```python
from build123d import *

# Parameters (mm, degrees)
SKETCH_1_W                = 33
SKETCH_1_H                = 6
EXTRUDE_1_DEPTH           = 30
SKETCH_3_R                = 6
EXTRUDE_2_DEPTH           = 10
SKETCH_4_R                = 3.1
CUT_EXTRUDE_1_DEPTH       = 15
SKETCH_5_R                = 1.75
CUT_EXTRUDE_2_DEPTH       = 48.053161424
EXTRUDE_3_REACH           = 49.381
EXTRUDE_3_END_RADIUS      = 6
SKETCH_10_R               = 1
HOLE_WIZARD_M4_7_D        = 3.3
HOLE_WIZARD_M4_7_DEPTH    = 15
HOLE_WIZARD_M4_7_TIP      = 0.991420021
EXTRUDE_4_REACH           = 49.381
EXTRUDE_4_END_RADIUS      = 6
SKETCH_17_R               = 1.5
HOLE_WIZARD_M4_8_D        = 3.3
HOLE_WIZARD_M4_8_DEPTH    = 13
HOLE_WIZARD_M4_8_TIP      = 0.991420021
HOLE_WIZARD_1_D           = 3.4
HOLE_WIZARD_1_CBORE_D     = 6
HOLE_WIZARD_1_CBORE_DEPTH = 3.4
CUT_EXTRUDE_3_DEPTH       = 46.70557955


with BuildPart() as part:
    # 草图1 → 凸台-拉伸1 (new body)
    with BuildSketch(Plane.XY):
        with Locations((16.5, -3)):
            Rectangle(SKETCH_1_W, SKETCH_1_H)
    extrude(amount=EXTRUDE_1_DEPTH)

    # 草图3 → 凸台-拉伸2 (add)
    with BuildSketch(Plane.XZ.offset(6)):
        with Locations(Location((10.6, 15, 0), (0, 0, 90))):
            Circle(SKETCH_3_R)
    extrude(amount=EXTRUDE_2_DEPTH)

    # 草图4 → 切除-拉伸1 (cut)
    with BuildSketch(Plane.XZ.offset(16)):
        with Locations(Location((10.6, 15, 0), (0, 0, 270))):
            Circle(SKETCH_4_R)
    extrude(amount=-CUT_EXTRUDE_1_DEPTH, mode=Mode.SUBTRACT)

    # 草图5 → 切除-拉伸2 (cut, through all)
    with BuildSketch(Plane.XZ.offset(1)):
        with Locations(Location((10.6, 15, 0), (0, 0, 270))):
            Circle(SKETCH_5_R)
    extrude(amount=-CUT_EXTRUDE_2_DEPTH, mode=Mode.SUBTRACT)

    # 凸台-拉伸3: up to this cylinder (the profile starts outside it)
    extrude_3_end = Plane(origin=(10.6, -11, 15), z_dir=(0, 1, 0)) * Cylinder(EXTRUDE_3_END_RADIUS, 111.762, mode=Mode.PRIVATE)
    # 草图10 → 凸台-拉伸3 (add, up to the surface)
    with BuildSketch(Plane.XY, mode=Mode.PRIVATE) as extrude_3_sk1:
        with Locations(Location((10.6, -11, 0), (0, 0, 180))):
            Circle(SKETCH_10_R)
    extrude_3_tool1 = extrude(extrude_3_sk1.sketch, amount=EXTRUDE_3_REACH, mode=Mode.PRIVATE) - extrude_3_end
    add(extrude_3_tool1.solids().sort_by_distance((10.6, -11, 0))[0])

    # M4 螺纹孔7
    with Locations(Plane(origin=(10.6, -11, 0), x_dir=(-1, 0, 0), z_dir=(0, 0, -1))):
        with Locations((0, 0)):
            Hole(HOLE_WIZARD_M4_7_D / 2, depth=HOLE_WIZARD_M4_7_DEPTH)
            with Locations((0, 0, -(HOLE_WIZARD_M4_7_DEPTH + HOLE_WIZARD_M4_7_TIP / 2))):  # 118° drill point
                Cone(0, HOLE_WIZARD_M4_7_D / 2, HOLE_WIZARD_M4_7_TIP, mode=Mode.SUBTRACT)

    # 凸台-拉伸4: up to this cylinder (the profile starts outside it)
    extrude_4_end = Plane(origin=(10.6, -11, 15), z_dir=(0, 1, 0)) * Cylinder(EXTRUDE_4_END_RADIUS, 111.762, mode=Mode.PRIVATE)
    # 草图17 → 凸台-拉伸4 (add, up to the surface)
    with BuildSketch(Plane(origin=(0, 0, 0), x_dir=(0, 0, -1), z_dir=(1, 0, 0)), mode=Mode.PRIVATE) as extrude_4_sk1:
        with Locations(Location((-15, -11, 0), (0, 0, 180))):
            Circle(SKETCH_17_R)
    extrude_4_tool1 = extrude(extrude_4_sk1.sketch, amount=EXTRUDE_4_REACH, mode=Mode.PRIVATE) - extrude_4_end
    add(extrude_4_tool1.solids().sort_by_distance((0, -11, 15))[0])

    # M4 螺纹孔8
    with Locations(Plane(origin=(0, -11, 15), x_dir=(0, 0, -1), z_dir=(-1, 0, 0))):
        with Locations((0, 0)):
            Hole(HOLE_WIZARD_M4_8_D / 2, depth=HOLE_WIZARD_M4_8_DEPTH)
            with Locations((0, 0, -(HOLE_WIZARD_M4_8_DEPTH + HOLE_WIZARD_M4_8_TIP / 2))):  # 118° drill point
                Cone(0, HOLE_WIZARD_M4_8_D / 2, HOLE_WIZARD_M4_8_TIP, mode=Mode.SUBTRACT)

    # 打孔尺寸(%根据)内六角圆柱头螺钉的类型1 (through all)
    with Locations(Plane(origin=(29, -6, 20), x_dir=(0, 0, -1), z_dir=(0, -1, 0))):
        with Locations((0, 0), (10, 0)):
            CounterBoreHole(HOLE_WIZARD_1_D / 2, HOLE_WIZARD_1_CBORE_D / 2, HOLE_WIZARD_1_CBORE_DEPTH)

    # 草图22 → 切除-拉伸3 (cut, through all)
    with BuildSketch(Plane.XZ.offset(6)):
        with BuildLine():
            Line((10.6, 21), (25, 21))
            Line((25, 21), (25, 30))
            Line((25, 30), (0, 30))
            Line((0, 30), (0, 0))
            Line((0, 0), (25, 0))
            Line((25, 0), (25, 9))
            Line((25, 9), (10.6, 9))
            ThreePointArc((10.6, 9), (4.6, 15), (10.6, 21))
        make_face()
    extrude(amount=-CUT_EXTRUDE_3_DEPTH, mode=Mode.SUBTRACT)


solid = part.part
```
Can you work these out from the model? Positions are in its coordinate system, mm. A direction names the side the tool comes from. Coordinates: 2 decimals unless noted, no trailing zeros. Loops run counter-clockwise (first coordinate to the right, second up) from the corner with the lowest first, then second, coordinate; pieces in that order, holes last.
Item 1: Which directions (+Z, -Z, +X, -X, +Y, -Y) give clear straight access to the entire face, cutting with the end or side of a thin tool? Please do faces 1 (the face through (18, -3, 21)), 2 (the face through (6.308, -10.368, 16.524)), 3 (the face through (25, -3, 4)), 4 (the face through (27.2, -4.3, 12.4)).
Answers below:
face 1: +Z, -X, +Y, -Y
face 2: -X
face 3: -Z, -X, +Y, -Y
face 4: -Y
Item 2: Suppose I cut it at D-D (z = 20). Please give me the cut outline in (x, y).
Answers below:
outline: (7.28, -16) - (13.92, -16) - (13.92, -6) - (26, -6) - (26, -2.6) - (27.3, -2.6) - (27.3, 0) - (7.28, 0) - close; (30.7, -2.6) - (32, -2.6) - (32, -6) - (33, -6) - (33, 0) - (30.7, 0) - close
Item 3: Suppose I cut it at C-C (z = 10.75). Please give me the cut outline in (x, y).
Answers below:
outline: (6.36, -16) - (14.84, -16) - (14.84, -6) - (26.1, -6) - (26.1, -2.6) - (27.47, -2.6) - (27.47, 0) - (6.36, 0) - close; (30.53, -2.6) - (31.9, -2.6) - (31.9, -6) - (33, -6) - (33, 0) - (30.53, 0) - close; hole circle Ø3.3 at (10.6, -11)
Item 4: Suppose I cut it at A-A (x = 29). Please give me the cut outline in (y, z), then the cut area to 3 significant figures.
Answers below:
outline: (-6, 0) - (0, 0) - (0, 8.3) - (-2.6, 8.3) - (-2.6, 7) - (-6, 7) - close; (-6, 13) - (-2.6, 13) - (-2.6, 11.7) - (0, 11.7) - (0, 18.3) - (-2.6, 18.3) - (-2.6, 17) - (-6, 17) - close; (-6, 23) - (-2.6, 23) - (-2.6, 21.7) - (0, 21.7) - (0, 30) - (-6, 30) - close
area: 122 mm2
Item 5: If we mould it in two halves opening along Z, with no side actions, what happens to faces 5 (the face through (33, -3, 15)), 6 (the face through (9.05, -0.51, 14.19)), 7 (the face through (18, -3, 9)), 8 (the face through (27, -2.6, 10))? For each: released by +Z, released by -Z, zero draft, split by the parting line, or undercut.
Answers below:
face 5: zero draft
face 6: undercut
face 7: released by -Z
face 8: undercut
Item 6: Suppose I cut it at B-B (y = -2). Please give me the cut outline in (x, z).
Answers below:
outline: (10.6, 9) - (25, 9) - (25, 0) - (33, 0) - (33, 30) - (25, 30) - (25, 21) - (10.6, 21) arc R6 ccw to start; hole circle Ø6.2 at (10.6, 15); hole circle Ø3.4 at (29, 10); hole circle Ø3.4 at (29, 20)
Item 7: I'm going to push flat-ended pins straight in: pin 1 (1.8 mm diameter, centred on x = 28.5, z = 20.5, fed in from -Y); pin 2 (5 mm diameter, centred on y = -4.5, z = 7, fed in from -X); pin 3 (6.5 mm diameter, centred on x = 15, y = -4.5, fed in from +Z); pin 4 (8 mm diameter, centred on x = 29, z = 10, fed in from +Y). Where does each tip first touch, or does it pass through?
Answers below:
pin 1: passes through
pin 2: stops at x = 8.2
pin 3: stops at z = 21
pin 4: stops at y = 0
Item 8: Please list where these lines run through material, in increasing order: L1, parallel to X at y = -8, z = 15; L2, parallel to X at y = -5.5, z = 20; L3, parallel to Y at x = 16.5, z = 11.25.
Answers below:
L1: x = 4.6 to 7.5, 13.7 to 16.6
L2: x = 7.28 to 26, 32 to 33
L3: y = -6 to 0
